Design review of the part built by this model. Coordinates are the model's own, in mm. A direction names the side the tool comes from. Coordinates: 2 decimals unless noted, no trailing zeros. Loops run counter-clockwise (first coordinate to the right, second up) from the corner with the lowest first, then second, coordinate; pieces in that order, holes last. Notation, with made-up numbers: M 11,43 L 28,43 A23 ccw 28,56 Z; hole C -13.75,33.25 d11. An arc over 180 degrees is marked long. Answer as a JSON object with one key per item and string values. Group by question number.
1. Draft analysis for pull direction Y (two halves, no side actions). For faces 1 (the flat face through (0, 6, -5)), 2 (the cylindrical face through (-2.539, -1.947, -2.465)), 3 (the flat face through (0, 27.5, -2)), state which applies: +Y half, -Y half, draft (parallel to the pull), parting line (faces both ways), or undercut.
2. Consider section D-D (y = 21). State the section outline as (x, z) points, then the cut area to 3 significant figures.
3. Consider section A-A (x = 0). State the section outline as (y, z) points, then the cut area to 3 significant figures.
4. Machinability: for faces 4 (the flat face through (-22, -17.5, -2)), 5 (the flat face through (17.5, -22, -2)), 6 (the flat face through (22, 17.5, -2)), 7 (the flat face through (0, -27.5, -2)), 8 (the flat face through (-23, 17.5, -2)), which of the approach directions +Z, -Z, +X, -X, +Y, -Y give a long, thin tool a straight path to every point of the face, cutting with its end or side? Answer none if there is none.
5. Insertion check: pin 1 (4 mm diameter, centred on x = 0.5, y = 5, fed in from +Z); pin 2 (1.5 mm diameter, centred on x = -21, z = -3, fed in from -Y); pin 3 (1.5 mm diameter, centred on y = 23, z = -3, fed in from -X); pin 4 (1.5 mm diameter, centred on y = -23.5, z = -1.5, fed in from +X). Each pin has a flat end and moves straight along its axis. Give the tip position at first contact, or say it passes through.
6. Consider section C-C (z = -1.95). State the section outline as (x, y) points, then the cut area to 3 significant figures.
7. To check wall thickness, follow probe 1 along Y at (x, z) = (0, -2.65); probe 2 along Y at (x, z) = (-23, -1.55); probe 3 along X at (y, z) = (0.5, -1.35). State the ranges of each line that lie inside material, in increasing order.
from build123d import *

# Parameters (mm, degrees)
SKETCH1_R           = 3.2
BOSS_EXTRUDE1_DEPTH = 5


with BuildPart() as part:
    # Sketch1 → Boss-Extrude1 (new body)
    with BuildSketch(Plane.XY):
        Polygon((-17.5, 27.5), (17.5, 27.5), (17.5, 17.5), (27.5, 17.5), (27.5, -17.5), (17.5, -17.5), (17.5, -27.5), (-17.5, -27.5), (-17.5, -17.5), (-27.5, -17.5), (-27.5, 17.5), (-17.5, 17.5), align=None)
        Circle(SKETCH1_R, mode=Mode.SUBTRACT)
    extrude(amount=-BOSS_EXTRUDE1_DEPTH)


solid = part.part
Findings below:
{
 "1": {"face 1": "draft", "face 2": "undercut", "face 3": "+Y half"},
 "2": {"outline": "M -17.5,-5 L 17.5,-5 L 17.5,0 L -17.5,0 Z", "area": "175 mm^2"},
 "3": {"outline": "M -27.5,-5 L -3.2,-5 L -3.2,0 L -27.5,0 Z; M 3.2,-5 L 27.5,-5 L 27.5,0 L 3.2,0 Z", "area": "243 mm^2"},
 "4": {"face 4": "+Z, -Z, -X, -Y", "face 5": "+Z, -Z, +X, -Y", "face 6": "+Z, -Z, +X, +Y", "face 7": "+Z, -Z, +X, -X, -Y", "face 8": "+Z, -Z, -X, +Y"},
 "5": {"pin 1": "stops at z = 0", "pin 2": "stops at y = -17.5", "pin 3": "stops at x = -17.5", "pin 4": "stops at x = 17.5"},
 "6": {"outline": "M -27.5,-17.5 L -17.5,-17.5 L -17.5,-27.5 L 17.5,-27.5 L 17.5,-17.5 L 27.5,-17.5 L 27.5,17.5 L 17.5,17.5 L 17.5,27.5 L -17.5,27.5 L -17.5,17.5 L -27.5,17.5 Z; hole C 0,0 d6.4", "area": "2,590 mm^2"},
 "7": {"probe 1": "y = -27.5 to -3.2, 3.2 to 27.5", "probe 2": "y = -17.5 to 17.5", "probe 3": "x = -27.5 to -3.16, 3.16 to 27.5"}
}
